Geometry: see drawing. Coordinates: mm, zero at the bounding-box minimum. A direction names the side the tool comes from. Coordinates: 2 decimals unless noted, no trailing zeros. Order: outer loops, then holes, each group sorted by start corner. A loop starts at its lowest first (then second) coordinate and runs counter-clockwise, first axis right, second up. Notation, with made-up numbers: M 70,-1 L 92,-1 A9 cw 92,16 Z; hole C -3.75,82.5 d9. An arc over 180 degrees is marked long. Answer in a Markdown table with one row per item.
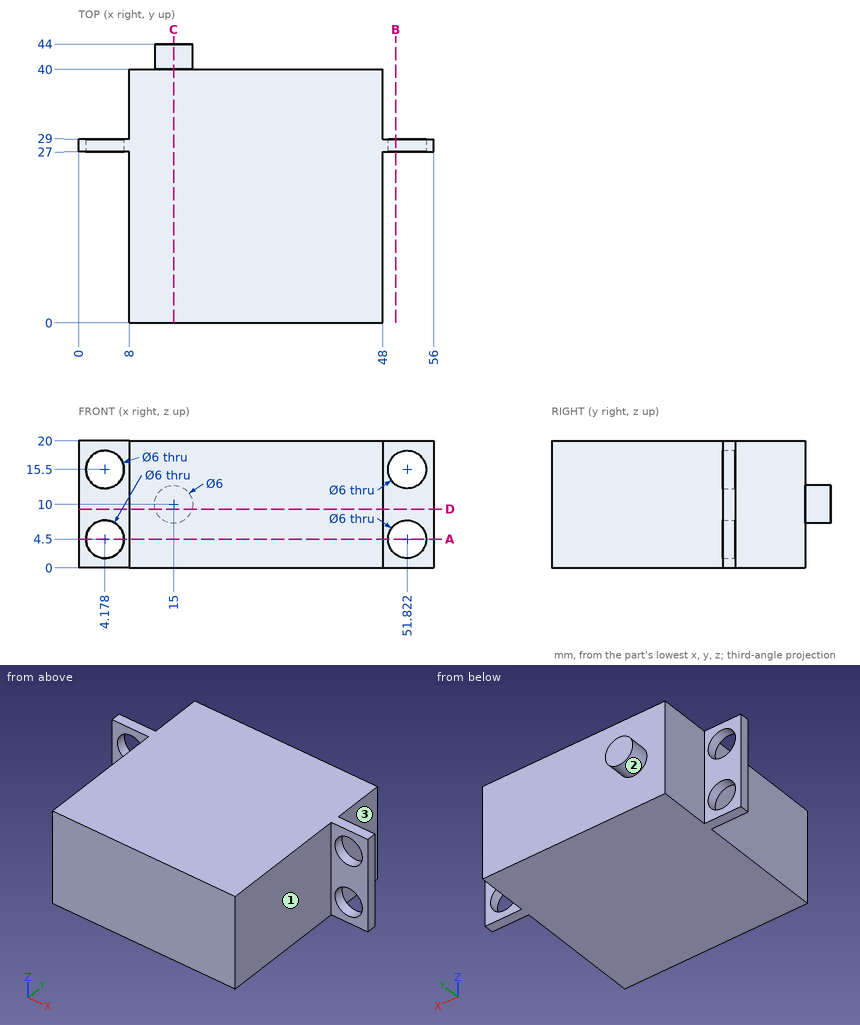
1) Reachability of the marked faces 1, 2 and 3 from +Z, -Z, +X, -X, +Y, -Y: full face, straight path, thin tool, end or side. Return the list, or none.
Resolved:
| item | result |
|---|---|
| face 1 | +Z, -Z, +X, -Y |
| face 2 | +Y |
| face 3 | +Z, -Z, +X, +Y |
2) Material intervals for probe 1 along X at (y, z) = (28.3, 4.5); probe 2 along Y at (x, z) = (9.5, 18); probe 3 along X at (y, z) = (18, 3), sorted ascending.
Resolved:
| item | result |
|---|---|
| probe 1 | x = 0 to 1.18, 7.18 to 48.82, 54.82 to 56 |
| probe 2 | y = 0 to 40 |
| probe 3 | x = 8 to 48 |
3) Cut plane B-B, the plane x = 50. Output: boundary loops of the cut face in (y, z).
Resolved:
| item | result |
|---|---|
| outline | M 27,0 L 29,0 L 29,2.12 L 27,2.12 Z; M 27,6.88 L 29,6.88 L 29,13.12 L 27,13.12 Z; M 27,17.88 L 29,17.88 L 29,20 L 27,20 Z |
4) Cut plane A-A, the plane z = 4.5. Output: boundary loops of the cut face in (x, y).
Resolved:
| item | result |
|---|---|
| outline | M 0,27 L 1.18,27 L 1.18,29 L 0,29 Z; M 7.18,27 L 8,27 L 8,0 L 48,0 L 48,27 L 48.82,27 L 48.82,29 L 48,29 L 48,40 L 8,40 L 8,29 L 7.18,29 Z; M 54.82,27 L 56,27 L 56,29 L 54.82,29 Z |
5) Cut plane D-D, the plane z = 9.25. Output: boundary loops of the cut face in (x, y).
Resolved:
| item | result |
|---|---|
| outline | M 0,27 L 8,27 L 8,0 L 48,0 L 48,27 L 56,27 L 56,29 L 48,29 L 48,40 L 17.9,40 L 17.9,44 L 12.1,44 L 12.1,40 L 8,40 L 8,29 L 0,29 Z |
6) Cut plane C-C, the plane x = 15. Output: boundary loops of the cut face in (y, z), and give its area (3 significant figures).
Resolved:
| item | result |
|---|---|
| outline | M 0,0 L 40,0 L 40,7 L 44,7 L 44,13 L 40,13 L 40,20 L 0,20 Z |
| area | 824 mm2 |
7) Contact query for flat-ended pins moving along their axis: pin 1 (9 mm diameter, centred on y = 37, z = 8, fed in from +X); pin 2 (2.5 mm diameter, centred on x = 4.5, z = 10, fed in from +Y); pin 3 (8 mm diameter, centred on x = 51.82, z = 15.5, fed in from +Y). Output: stop coordinate, or through.
Resolved:
| item | result |
|---|---|
| pin 1 | stops at x = 48 |
| pin 2 | stops at y = 29 |
| pin 3 | stops at y = 40 |
